Geometry: final body of the model. Coordinates: model frame, mm. Face numbers are marked on the shaded views. Coordinates: 2 decimals unless noted, no trailing zeros. Loops run counter-clockwise (first coordinate to the right, second up) from the corner with the lowest first, then second, coordinate; pieces in that order, holes last. Notation, with made-up numbers: (65.25, 26.5) - (88.25, 26.5) arc R16 cw to (88.25, 48.5) - close; hole circle Ø3 at (-0.5, -0.75). An arc over 180 degrees is marked (long way). Return JSON: item names as keys, results as strings.
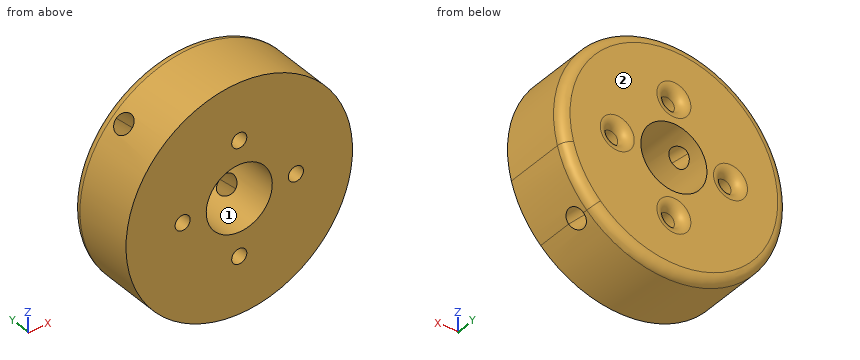
from build123d import *

# Parameters (mm, degrees)
SKETCH1_R           = 24
SKETCH1_R_2         = 7
SKETCH1_R_3         = 1.6
BOSS_EXTRUDE1_DEPTH = 15
BOSS_EXTRUDE2_START = -16
BOSS_EXTRUDE2_DEPTH = 16
CUT_EXTRUDE1_DEPTH  = 72
CUT_EXTRUDE2_START  = -72
CUT_EXTRUDE2_DEPTH  = 72
FILLET3_R           = 2


with BuildPart() as part:
    # Sketch1 → Boss-Extrude1 (new body)
    with BuildSketch(Plane(origin=(0, 0, 0), x_dir=(1, 0, 0), z_dir=(0, 1, 0))):
        with Locations(Location((0, 0, 0), (0, 0, 270))):
            Circle(SKETCH1_R)
        with Locations(Location((0, 0, 0), (0, 0, 270))):
            Circle(SKETCH1_R_2, mode=Mode.SUBTRACT)
        with Locations(Location((0, 12, 0), (0, 0, 270))):
            Circle(SKETCH1_R_3, mode=Mode.SUBTRACT)
        with Locations(Location((12, 0, 0), (0, 0, 270))):
            Circle(SKETCH1_R_3, mode=Mode.SUBTRACT)
        with Locations(Location((0, -12, 0), (0, 0, 270))):
            Circle(SKETCH1_R_3, mode=Mode.SUBTRACT)
        with Locations(Location((-12, 0, 0), (0, 0, 270))):
            Circle(SKETCH1_R_3, mode=Mode.SUBTRACT)
    extrude(amount=BOSS_EXTRUDE1_DEPTH)

    # Sketch3 → Boss-Extrude2 (add)
    with BuildSketch(Plane(origin=(0, 15, 0), x_dir=(1, 0, 0), z_dir=(0, 1, 0)).offset(BOSS_EXTRUDE2_START)):
        with BuildLine():
            Line((16.970562748, 16.970562748), (25.455844123, 8.485281374))
            Line((25.455844123, 8.485281374), (23.182219831, 6.211657082))
            ThreePointArc((23.182219831, 6.211657082), (20.784609691, 12), (16.970562748, 16.970562748))
        make_face()
    extrude(amount=BOSS_EXTRUDE2_DEPTH)

    # Sketch4 → Cut-Extrude1 (cut)
    with BuildSketch(Plane(origin=(16.970562748, 0, -16.970562748), x_dir=(-0.7071067811865489, 0, -0.7071067811865461), z_dir=(0.7071067811865461, 0, -0.7071067811865489))):
        with BuildLine():
            ThreePointArc((0, 12.1), (-2.1, 10), (0, 7.9))
            Line((0, 7.9), (0, 10))
            Line((0, 10), (0, 12.1))
        make_face()
        with BuildLine():
            Line((0, 10), (0, 7.9))
            ThreePointArc((0, 7.9), (1.48492424, 8.51507576), (2.1, 10))
            ThreePointArc((2.1, 10), (1.48492424, 11.48492424), (0, 12.1))
            Line((0, 12.1), (0, 10))
        make_face()
    extrude(amount=-CUT_EXTRUDE1_DEPTH, mode=Mode.SUBTRACT)

    # Sketch5 → Cut-Extrude2 (cut)
    with BuildSketch(Plane(origin=(0, 15, 0), x_dir=(1, 0, 0), z_dir=(0, 1, 0)).offset(CUT_EXTRUDE2_START)):
        with BuildLine():
            Line((23.182219831, 6.211657082), (25.455844123, 8.485281374))
            Line((25.455844123, 8.485281374), (16.970562748, 16.970562748))
            ThreePointArc((16.970562748, 16.970562748), (20.784609691, 12), (23.182219831, 6.211657082))
        make_face()
    extrude(amount=CUT_EXTRUDE2_DEPTH, mode=Mode.SUBTRACT)

    # Fillet3
    fillet3_edges = [part.edges().sort_by_distance(p)[0] for p in [
        (12, 15, -1.6),
        (0, 15, 10.4),
        (-12, 15, -1.6),
        (-20.784609691, 15, 12),
        (0, 15, -13.6),
    ]]
    fillet(fillet3_edges, radius=FILLET3_R)


solid = part.part
Item 1: First-contact query: pin 1 Ø4 at (y, z) = (4, -5) entering from +X; pin 2 Ø6 at (x, y) = (18.5, 12) entering from +Z; pin 3 Ø5 at (x, z) = (12, 0) entering from +Y; pin 4 Ø3 at (x, z) = (0, -12) entering from -Y. Flat tips, straight axial feed; report the tip coordinate or a pass-through.
Worked out:
{"pin 1": "x = 23.81", "pin 2": "z = 18.32", "pin 3": "y = 14.67", "pin 4": "through"}
Item 2: Mould query, pull axis Z, two halves, no side actions, for the marked faces 1 and 2. Classes: +Z half, -Z half, draft (parallel to the pull), parting line (faces both ways), or undercut.
Worked out:
{"face 1": "undercut", "face 2": "draft"}
Item 3: Section query A-A, the plane z = 0. Return loops of the section in (x, y).
Worked out:
{"outline": "(-24, 0) - (-13.6, 0) - (-13.6, 13) arc R2 ccw to (-15.6, 15) - (-22, 15) arc R2 ccw to (-24, 13) - close; (-10.4, 0) - (-7, 0) - (-7, 15) - (-8.4, 15) arc R2 ccw to (-10.4, 13) - close; (7, 0) - (10.4, 0) - (10.4, 13) arc R2 ccw to (8.4, 15) - (7, 15) - close; (13.6, 0) - (24, 0) - (24, 13) arc R2 ccw to (22, 15) - (15.6, 15) arc R2 ccw to (13.6, 13) - close"}
Item 4: Section query B-B, the plane x = 0. Return loops of the section in (y, z), and give its area (3 significant figures).
Worked out:
{"outline": "(0, -24) - (13, -24) arc R2 ccw to (15, -22) - (15, -15.6) arc R2 ccw to (13, -13.6) - (0, -13.6) - close; (0, -10.4) - (13, -10.4) arc R2 ccw to (15, -8.4) - (15, -7) - (0, -7) - close; (0, 7) - (15, 7) - (15, 8.4) arc R2 ccw to (13, 10.4) - (0, 10.4) - close; (0, 13.6) - (13, 13.6) arc R2 ccw to (15, 15.6) - (15, 22) arc R2 ccw to (13, 24) - (0, 24) - close", "area": "409 mm^2"}
Item 5: Ray query, probe 1 along X at (y, z) = (11.5, -13); probe 2 along X at (y, z) = (9, 11.5); probe 3 along X at (y, z) = (1.75, 0.5). Return the intervals inside material, ascending. Write a range as from..to.
Worked out:
{"probe 1": "-20.17..-1.25, 1.25..10.92, 15.08..20.17", "probe 2": "-21.07..-14.11, -8.89..-1.52, 1.52..21.07", "probe 3": "-23.99..-13.52, -10.48..-6.98, 6.98..10.48, 13.52..23.99"}
Item 6: Section query C-C, the plane y = 6.5. Return loops of the section in (x, z), and give its area (3 significant figures).
Worked out:
{"outline": "circle Ø48 at (0, 0); hole circle Ø3.2 at (-12, 0); hole circle Ø14 at (0, 0); hole circle Ø3.2 at (0, -12); hole circle Ø3.2 at (0, 12); hole circle Ø3.2 at (12, 0)", "area": "1,620 mm^2"}
Item 7: Section query D-D, the plane y = 11.5. Return loops of the section in (x, z).
Worked out:
{"outline": "(-17.98, 15.9) arc R24 ccw to (15.9, -17.98) - (3.8, -5.88) arc R7 cw to (-5.88, 3.8) - close; (-15.9, 17.98) - (-3.8, 5.88) arc R7 cw to (5.88, -3.8) - (17.98, -15.9) arc R24 ccw to start; hole circle Ø3.2 at (-12, 0); hole circle Ø3.2 at (0, -12); hole circle Ø3.2 at (0, 12); hole circle Ø3.2 at (12, 0)"}
